Geometry check sheet. Reference: the model listing, model coordinates, mm. Coordinates: 2 decimals unless noted, no trailing zeros. Order: outer loops, then holes, each group sorted by start corner. A loop starts at its lowest first (then second) coordinate and runs counter-clockwise, first axis right, second up. Notation, with made-up numbers: (49, -35.75) -> (99, -35.75) arc R24 ccw to (99, -6.75) -> close; hole circle Ø6 at (12, 83.5). An arc over 180 degrees is marked (long way). Answer as CSV lines item,"result". Start each with the question number.
Autodesk Inventor part; units mm, degrees
ref_plane "YZ Plane" through (0, 0, 0) normal (1, 0, 0) x (0, 1, 0)
ref_plane "XZ Plane" through (0, 0, 0) normal (0, 1, 0) x (-1, 0, 0)
ref_plane "XY Plane" through (0, 0, 0) normal (0, 0, 1) x (1, 0, 0)
sketch "Sketch1" plane through (0, 0, 0) normal (0, 0, 1) x (1, 0, 0)
  circle A0 centre (0, 0) radius 0.5
  line L0 (-3, 97) -> (3, 97)
  line L1 (5, 95) -> (5, -1)
  line L2 (3, -3) -> (-3, -3)
  line L3 (-5, -1) -> (-5, 95)
  arc A1 (-3, 97) -> (-5, 95) centre (-3, 95) ccw
  arc A2 (5, 95) -> (3, 97) centre (3, 95) ccw
  arc A3 (-5, -1) -> (-3, -3) centre (-3, -1) ccw
  arc A4 (3, -3) -> (5, -1) centre (3, -1) ccw
  circle A5 centre (0, 92) radius 2.5
  line L4 (0, 97) -> (0, 86.8445)
  circle A6 centre (-3.25, 0) radius 0.5
  circle A7 centre (3.25, 0) radius 0.5
  point P0 (-5, 97)
  point P1 (-5, -3)
  point P2 (0, -3)
  dimension "d3" = 1
  dimension "d7" = 100
  dimension "d8" = 10
  dimension "d9" = 3
  dimension "d10" = 2
  dimension "d11" = 5
  dimension "d12" = 5
  dimension "d15" = 1
  dimension "d16" = 1
  dimension "d17" = 3.25
  dimension "d18" = 3.25
extrude "Extrusion1" add sketch "Sketch1" along normal blind 3
properties part number "FP V2 Servo Arm v2"
Q1. Sectioned sample at A-A, the plane y = 92. Record the cut outline in (x, z), then the cut area to 3 significant figures.
Q2. Release check for a two-part mould opening along X. For faces 1 (the cylindrical face through (-0.33, 89.52, 1.48)), 2 (the flat face through (0, 48, 0)), 3 (the cylindrical face through (-4.4, -2.43, 1.48)) record: released by +X, released by -X, zero draft, split by the parting line, or undercut.
Q3. Thickness scan on L1, parallel to Y at x = 0, z = 0.65; L2, parallel to Y at x = 3.25, z = 2.2; L3, parallel to Y at x = 1.5, z = 1.15. Record the ranges inside material, lowest first.
Q4. Sectioned sample at C-C, the plane z = 1.95. Record the cut outline in (x, y).
Q5. Go/stop test with a flat-tipped pin: pin 1 Ø6 at (x, y) = (-3, 17.5) entering from -Z. Record where the tip stops, or that it passes through.
Q6. Sectioned sample at B-B, the plane x = 1.5. Record the cut outline in (y, z), then the cut area to 3 significant figures.
Geometry results:
1,outline,"(-5, 0) -> (-2.5, 0) -> (-2.5, 3) -> (-5, 3) -> close; (2.5, 0) -> (5, 0) -> (5, 3) -> (2.5, 3) -> close"
1,area,"15.0 mm^2"
2,face 1,"undercut"
2,face 2,"zero draft"
2,face 3,"released by -X"
3,L1,"y = -3 to -0.5, 0.5 to 89.5, 94.5 to 97"
3,L2,"y = -2.98 to -0.5, 0.5 to 96.98"
3,L3,"y = -3 to 90, 94 to 97"
4,outline,"(-5, -1) arc R2 ccw to (-3, -3) -> (3, -3) arc R2 ccw to (5, -1) -> (5, 95) arc R2 ccw to (3, 97) -> (-3, 97) arc R2 ccw to (-5, 95) -> close; hole circle Ø1 at (-3.25, 0); hole circle Ø5 at (0, 92); hole circle Ø1 at (0, 0); hole circle Ø1 at (3.25, 0)"
5,pin 1,"stops at z = 0"
6,outline,"(-3, 0) -> (90, 0) -> (90, 3) -> (-3, 3) -> close; (94, 0) -> (97, 0) -> (97, 3) -> (94, 3) -> close"
6,area,"288 mm^2"
